Work out the finished part from the listing and answer in its coordinate system (mm). A direction names the side the tool comes from. Round coordinates to 2 decimals unless told otherwise and drop trailing zeros. Write each loop counter-clockwise with the first axis right and the second up, starting at its lowest first coordinate (ties: lowest second). Pieces come first, ordered by that corner, then holes.
1. Flat-ended cylindrical pins translate along their axes: pin 1 Ø12 at (y, z) = (21.5, -0.5) entering from -X; pin 2 Ø3 at (x, z) = (31.5, -4) entering from +Y; pin 3 Ø4.5 at (x, z) = (35, -3) entering from -Y; pin 4 Ø2.5 at (x, y) = (32.5, 1) entering from +Z. Find the tip coordinate at first contact, or state that the pin passes through.
2. Find section A-A (z = -3). Write down the section's boundary in (x, y), and give its area (3 significant figures).
3. A tool of negligible diameter and unlimited length cuts with its end or side. For faces 1 (the face through (5, 1, -6)), 2 (the face through (33, 1, 0)), 3 (the face through (38, 1, -3)), 4 (the face through (33, 1, -6)), from which of +Z, -Z, +X, -X, +Y, -Y can it reach the whole face along a straight path? Write none if from no direction.
4. Straight lines are drawn through the part: probe 1 along X at (y, z) = (14, -3); probe 2 along Z at (x, y) = (3, 1.1); probe 3 along X at (y, z) = (8.75, -1.75). For each, find the intervals that lie inside material, in ascending order.
5. Find section B-B (x = 19). Write down the section's boundary in (y, z).
6. Determine the mould class of faces 5 (the face through (5, 1, 0)), 6 (the face through (21.4, 12.32, 4.63)), 7 (the face through (22.9, 0, -10.3)), 8 (the face through (1.38, 1.48, -3.51)) for opening direction Z: pulls with the +Z half, pulls with the -Z half, needs draft (parallel to the pull), parting line crosses it, or undercut.
7. Find section D-D (y = 9.25). Write down the section's boundary in (x, z).
8. Find section C-C (z = -8). Write down the section's boundary in (x, y) (3 decimals), and give its area (3 significant figures).
```python
from build123d import *

# Parameters (mm, degrees)
BOSS_EXTRUDE1_DEPTH   = 3
BOSS_EXTRUDE1_2_DEPTH = 3
SKETCH1_3_R           = 10
SKETCH1_3_R_2         = 8
BOSS_EXTRUDE2_DEPTH   = 25
M3_CLEARANCE_HOLE1_D  = 3.4


with BuildPart() as part:
    # Sketch1 → Boss-Extrude1 (new body)
    with BuildSketch(Plane(origin=(0, 0, 0), x_dir=(1, 0, 0), z_dir=(0, 1, 0))):
        with BuildLine():
            ThreePointArc((29, 3), (28.884177258, 1.482423007), (28.539392014, 0))
            Line((28.539392014, 0), (38, 0))
            Line((38, 0), (38, 6))
            Line((38, 6), (28.539392014, 6))
            ThreePointArc((28.539392014, 6), (28.884177258, 4.517576993), (29, 3))
        make_face()
    extrude(amount=BOSS_EXTRUDE1_DEPTH)



with BuildPart() as body_2:
    # Sketch1 → Boss-Extrude1 2 (new body)
    with BuildSketch(Plane(origin=(0, 0, 0), x_dir=(1, 0, 0), z_dir=(0, 1, 0))):
        with BuildLine():
            Line((0, 0), (9.460607986, 0))
            ThreePointArc((9.460607986, 0), (9, 3), (9.460607986, 6))
            Line((9.460607986, 6), (0, 6))
            Line((0, 6), (0, 0))
        make_face()
    extrude(amount=BOSS_EXTRUDE1_2_DEPTH)


with BuildPart() as part_1:
    add(part.part)

    add(body_2.part)  # Boss-Extrude2 merges body 2
    # Sketch1_3 → Boss-Extrude2 (add)
    with BuildSketch(Plane(origin=(0, 0, 0), x_dir=(1, 0, 0), z_dir=(0, 1, 0))):
        with Locations(Location((19, 3, 0), (0, 0, 162.542396876))):
            Circle(SKETCH1_3_R)
        with Locations(Location((19, 3, 0), (0, 0, 270))):
            Circle(SKETCH1_3_R_2, mode=Mode.SUBTRACT)
    extrude(amount=BOSS_EXTRUDE2_DEPTH)

    # M3 Clearance Hole1 (through all)
    with Locations(Plane(origin=(0, 3, 0), x_dir=(1, 0, 0), z_dir=(0, 1, 0))):
        with Locations((3, 3), (35, 3)):
            Hole(M3_CLEARANCE_HOLE1_D / 2)


solid = part_1.part
```
Worked answers:
1. pin 1: stops at x = 9
1. pin 2: stops at y = 3
1. pin 3: stops at y = 0
1. pin 4: stops at z = 0
2. outline: (0, 0) - (1.3, 0) - (1.3, 3) - (0, 3) - close; (4.7, 0) - (11, 0) - (11, 25) - (9, 25) - (9, 3) - (4.7, 3) - close; (27, 0) - (33.3, 0) - (33.3, 3) - (29, 3) - (29, 25) - (27, 25) - close; (36.7, 0) - (38, 0) - (38, 3) - (36.7, 3) - close
2. area: 134 mm2
3. face 1: -Z, -X, +Y, -Y
3. face 2: +Z, +X, +Y, -Y
3. face 3: +Z, -Z, +X, +Y, -Y
3. face 4: -Z, +X, +Y, -Y
4. probe 1: x = 9 to 11, 27 to 29
4. probe 2: z = -6 to -4.7, -1.3 to 0
4. probe 3: x = 9.08 to 11.1, 26.9 to 28.92
5. outline: (0, -13) - (25, -13) - (25, -11) - (0, -11) - close; (0, 5) - (25, 5) - (25, 7) - (0, 7) - close
6. face 5: pulls with the +Z half
6. face 6: undercut
6. face 7: needs draft
6. face 8: undercut
7. outline: circle Ø20 at (19, -3); hole circle Ø16 at (19, -3)
8. outline: (10.34, 0) - (12.755, 0) - (12.755, 25) - (10.34, 25) - close; (25.245, 0) - (27.66, 0) - (27.66, 25) - (25.245, 25) - close
8. area: 121 mm2
